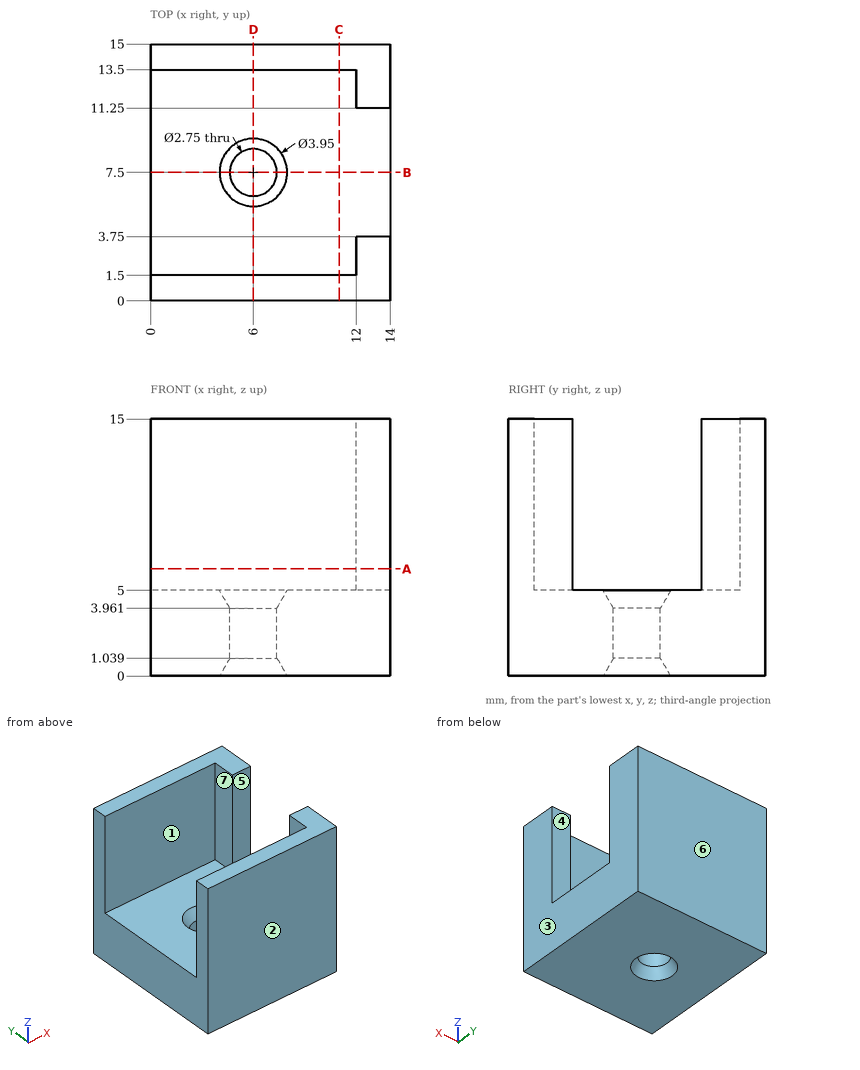
Job drawing, mm, ordinate dimensions from the low corner. One solid piece. A direction names the side the tool comes from. Give positions to 0.01 mm unless a question says otherwise; leave off trailing zeros. Write each loop counter-clockwise with the first axis right and the second up, starting at its lowest first coordinate (ties: lowest second). Pieces come first, ordered by that corner, then holes. Notation, with made-up numbers: M 35,9 L 45,9 A20 ccw 45,18 Z; hole C 72,89.25 d4. An arc over 180 degrees is marked long. One line per item, written item: value. Start each with the question number.
Q1. Saw through at C-C, the plane x = 11. Write the cut outline in (y, z).
Q2. Saw through at A-A, the plane z = 6.25. Write the cut outline in (x, y), plus the area to 3 significant figures.
Q3. Saw through at D-D, the plane x = 6. Write the cut outline in (y, z) (1 decimal), plus the area to 3 significant figures.
Q4. 3-axis set-ups, long thin cutter, end or side, ignore diameter. For the marked faces 5, 6 and 7: which of +Z, -Z, +X, -X, +Y, -Y reach the whole face in a straight line?
Q5. Probe probe 1 along Y at (x, z) = (4.75, 13.25); probe 2 along Y at (x, z) = (6, 2.2) (3 decimals); probe 3 along X at (y, z) = (7.5, 2.25) (3 decimals). List the from-to ranges inside material, lowest first. Write a range as [from, to].
Q6. Drop flat-ended pins along their axis: pin 1 Ø8 at (x, z) = (8, 4) entering from -Y; pin 2 Ø3.5 at (x, y) = (6, 7.5) entering from -Z; pin 3 Ø3 at (x, y) = (9.5, 11.5) entering from +Z. Give the stop position or say it passes through.
Q7. Saw through at B-B, the plane y = 7.5. Write the cut outline in (x, z) (1 decimal), plus the area to 3 significant figures.
Q8. Two-plate mould, pull along Y, no slides. Class the marked faces 1, 2, 3 and 4: +Y half, -Y half, draft (parallel to the pull), parting line (faces both ways), or undercut.
Output values:
1. outline: M 0,0 L 15,0 L 15,15 L 13.5,15 L 13.5,5 L 1.5,5 L 1.5,15 L 0,15 Z
2. outline: M 0,0 L 14,0 L 14,3.75 L 12,3.75 L 12,1.5 L 0,1.5 Z; M 0,13.5 L 12,13.5 L 12,11.25 L 14,11.25 L 14,15 L 0,15 Z
2. area: 51.0 mm²
3. outline: M 0,0 L 5.5,0 L 6.1,1 L 6.1,4 L 5.5,5 L 1.5,5 L 1.5,15 L 0,15 Z; M 8.9,1 L 9.5,0 L 15,0 L 15,15 L 13.5,15 L 13.5,5 L 9.5,5 L 8.9,4 Z
3. area: 90.0 mm²
4. face 5: +Z, +X, -X
4. face 6: +Z, -Z, +X, -X, +Y
4. face 7: +Z, -X
5. probe 1: y = [0, 1.5], [13.5, 15]
5. probe 2: y = [0, 6.125], [8.875, 15]
5. probe 3: x = [0, 4.625], [7.375, 14]
6. pin 1: stops at y = 0
6. pin 2: stops at z = 0.39
6. pin 3: stops at z = 5
7. outline: M 0,0 L 4,0 L 4.6,1 L 4.6,4 L 4,5 L 0,5 Z; M 7.4,1 L 8,0 L 14,0 L 14,5 L 8,5 L 7.4,4 Z
7. area: 55.0 mm²
8. face 1: undercut
8. face 2: -Y half
8. face 3: draft
8. face 4: undercut
